Build history of the part. All positions in model axes, mm. A direction names the side the tool comes from. Round coordinates to 2 decimals unless told otherwise and drop trailing zeros. Loops run counter-clockwise (first coordinate to the right, second up) from the corner with the lowest first, then second, coordinate; pieces in that order, holes last. Notation, with made-up numbers: (46, 1.25) - (82, 1.25) arc R33 cw to (82, 31.25) - close; hole circle Ø4 at (-11, 87). An arc over 180 degrees is marked (long way). Put each result on its own line as item: value. Start each with the question number.
from build123d import *

# Parameters (mm, degrees)
BOSS_EXTRUDE1_DEPTH = 5.4102


with BuildPart() as part:
    # Sketch1 → Boss-Extrude1 (new body)
    with BuildSketch(Plane.XY):
        Polygon((-165.481, 56.680227), (-165.481, 0), (165.481, 0), (165.481, 56.680227), (114.681, 56.680227), (114.681, 51.270027), (63.881, 51.270027), (63.881, 56.680227), (-63.881, 56.680227), (-63.881, 51.270027), (-114.681, 51.270027), (-114.681, 56.680227), align=None)
        Polygon((-165.481, 0), (-165.481, -56.680227), (-114.681, -56.680227), (-114.681, -51.270027), (-63.881, -51.270027), (-63.881, -56.680227), (63.881, -56.680227), (63.881, -51.270027), (114.681, -51.270027), (114.681, -56.680227), (165.481, -56.680227), (165.481, 0), align=None)
    extrude(amount=BOSS_EXTRUDE1_DEPTH)


solid = part.part
1) Pull direction X, two halves, no side cores. Call faces 4 (the face through (-165.481, 1, 3)), 5 (the face through (140, -56.68, 3)), 6 (the face through (90, 51.27, 3)), 7 (the face through (-114.681, -54, 3)): pulls with the +X half, pulls with the -X half, needs draft (parallel to the pull), parting line crosses it, or undercut.
2) Drill centre line: line 1 (Y direction, x = -98.5, z = 4.7). Where is it in solid material? Low to high. Write a range as [from, to].
3) Which spindle directions (+Z, -Z, +X, -X, +Y, -Y) get a long thin tool onto all of the face, cutting with end or side? Do faces 1 (the face through (165.481, -1, 3)), 2 (the face through (-114.681, 54, 3)), 3 (the face through (114.681, -54, 3)). Say none if no direction does.
4) Slice it at A-A, the plane z = 2. Write the cut outline in (x, y).
5) Drop flat-ended pins along their axis: pin 1 Ø2.5 at (x, z) = (80, 1.5) entering from +Y; pin 2 Ø1.6 at (x, z) = (81, 1.5) entering from -Y. Give the stop position or say it passes through.
6) Slice it at B-B, the plane x = -73.5. Write the cut outline in (y, z).
Taken from the geometry:
1. face 4: pulls with the -X half
1. face 5: needs draft
1. face 6: undercut
1. face 7: undercut
2. line 1: y = [-51.27, 51.27]
3. face 1: +Z, -Z, +X, +Y, -Y
3. face 2: +Z, -Z, +Y
3. face 3: +Z, -Z, -Y
4. outline: (-165.48, -56.68) - (-114.68, -56.68) - (-114.68, -51.27) - (-63.88, -51.27) - (-63.88, -56.68) - (63.88, -56.68) - (63.88, -51.27) - (114.68, -51.27) - (114.68, -56.68) - (165.48, -56.68) - (165.48, 56.68) - (114.68, 56.68) - (114.68, 51.27) - (63.88, 51.27) - (63.88, 56.68) - (-63.88, 56.68) - (-63.88, 51.27) - (-114.68, 51.27) - (-114.68, 56.68) - (-165.48, 56.68) - close
5. pin 1: stops at y = 51.27
5. pin 2: stops at y = -51.27
6. outline: (-51.27, 0) - (51.27, 0) - (51.27, 5.41) - (-51.27, 5.41) - close
